The listing builds one solid part. Answer for the finished solid, in the listing's coordinates (mm). A direction names the side the tool comes from. Give positions to 0.01 mm unless a question says otherwise; leave off trailing zeros. Order: outer loops, then holes, each group sorted by start corner. A loop starts at its lowest first (then second) coordinate and runs counter-clockwise, first axis right, second up. Notation, with made-up numbers: (-26, 76) - (27, 76) arc R5 cw to (27, 84) - close; hole circle Ø5 at (1, -33.75). An arc over 180 degrees is marked (long way). Use CSV: the item, a comma, the result in double quotes.
```python
from build123d import *

# Parameters (mm, degrees)
SKETCH1_W           = 24
SKETCH1_H           = 9
BOSS_EXTRUDE1_DEPTH = 5.7
FILLET1_R           = 4
FILLET2_R           = 4
CUT_EXTRUDE2_DEPTH  = 1
LPATTERN1_COUNT     = 2
LPATTERN1_PITCH     = 4


with BuildPart() as part:
    # Sketch1 → Boss-Extrude1 (new body)
    with BuildSketch(Plane(origin=(0, 0, 0), x_dir=(1, 0, 0), z_dir=(0, 1, 0))):
        with Locations((12, 4.5)):
            Rectangle(SKETCH1_W, SKETCH1_H)
    extrude(amount=BOSS_EXTRUDE1_DEPTH)

    # Fillet1
    fillet1_edges = [part.edges().sort_by_distance(p)[0] for p in [
        (0, 2.85, 0),
    ]]
    fillet(fillet1_edges, radius=FILLET1_R)

    # Fillet2
    fillet2_edges = [part.edges().sort_by_distance(p)[0] for p in [
        (0, 2.85, -9),
    ]]
    fillet(fillet2_edges, radius=FILLET2_R)

    # Sketch2 → Cut-Extrude2 (cut)
    with BuildSketch(Plane(origin=(0, 5.7, 0), x_dir=(1, 0, 0), z_dir=(0, 1, 0))):
        Polygon((12.767766953, 1.5), (11, 1.5), (8, 4.5), (11, 7.5), (12.767766953, 7.5), (9.767766953, 4.5), align=None)
    cut_extrude2 = extrude(amount=-CUT_EXTRUDE2_DEPTH, mode=Mode.SUBTRACT)

    # LPattern1: Cut-Extrude2 ×2
    with Locations(*[(i * LPATTERN1_PITCH, 0, 0) for i in range(1, LPATTERN1_COUNT)]):
        add(cut_extrude2, mode=Mode.SUBTRACT)


solid = part.part
```
Item 1: The part is cut by section A-A (x = 8.5). Give the vertices of the cut face in (y, z), and give its area (3 significant figures).
Taken from the geometry:
outline,"(0, -9) - (5.7, -9) - (5.7, -5) - (4.7, -5) - (4.7, -4) - (5.7, -4) - (5.7, 0) - (0, 0) - close"
area,"50.3 mm^2"
Item 2: Which of the six approach directions +Z, -Z, +X, -X, +Y, -Y give full straight-line access (tool end or side, diameter ignored) to faces 1 (the face through (1.141, 2.89, -7.797)), 2 (the face through (11.25, 5.21, -3.02))?
Taken from the geometry:
face 1,"-Z, -X, +Y, -Y"
face 2,"+Y"
Item 3: The mould has two halves that part along Z. Classify faces 3 (the face through (12, 5.7, -5)), 4 (the face through (14, 3, -9)), 5 (the face through (10, 4.7, -4)): +Z half, -Z half, draft (parallel to the pull), parting line (faces both ways), or undercut.
Taken from the geometry:
face 3,"draft"
face 4,"-Z half"
face 5,"undercut"
Item 4: The part is cut by section C-C (z = -2). Give the vertices of the cut face in (x, y).
Taken from the geometry:
outline,"(0.54, 0) - (24, 0) - (24, 5.7) - (16.27, 5.7) - (16.27, 4.7) - (14.5, 4.7) - (14.5, 5.7) - (12.27, 5.7) - (12.27, 4.7) - (10.5, 4.7) - (10.5, 5.7) - (0.54, 5.7) - close"
Item 5: Find the intervals of material crossed by line 1 along X through (y, z) = (5.3, -6.25); line 2 along Z through (x, y) = (9, 4.9); line 3 along X through (y, z) = (3.15, -5.75), in increasing order.
Taken from the geometry:
line 1,"0.2 to 9.75, 11.52 to 13.75, 15.52 to 24"
line 2,"-9 to -5.5, -3.5 to 0"
line 3,"0.07 to 24"
Item 6: The part is cut by section B-B (y = 2.05). Give the vertices of the cut face in (x, z).
Taken from the geometry:
outline,"(0, -5) arc R4 ccw to (4, -9) - (24, -9) - (24, 0) - (4, 0) arc R4 ccw to (0, -4) - close"
Item 7: The part is cut by section D-D (x = 13). Give the vertices of the cut face in (y, z), and give its area (3 significant figures).
Taken from the geometry:
outline,"(0, -9) - (5.7, -9) - (5.7, -5.5) - (4.7, -5.5) - (4.7, -3.5) - (5.7, -3.5) - (5.7, 0) - (0, 0) - close"
area,"49.3 mm^2"
